Read the model definition and answer for the solid it produces. Units are mm, in the model's axes. A direction names the side the tool comes from. Give positions to 0.01 mm unless a question says otherwise; leave off trailing zeros. Loops run counter-clockwise (first coordinate to the right, second up) from the corner with the lowest first, then second, coordinate; pieces in that order, holes last.
(1) Each of these flat-tipped pins is pushed along its axis until it touches: P1, Ø6.5, axis at y = 0, z = 57, coming from the +X side; P2, Ø1.7, axis at y = 1.5, z = 68.5, coming from the -X side; P3, Ø3, axis at x = 0, z = 4, coming from the +Y side. Where does it stop, or does it pass through?
(2) Determine the mould class of faces 1 (the face through (-2, 2, -77)), 2 (the face through (-3.9, 0, -9)), 3 (the face through (8.201, 4, 1)) for opening direction X: pulls with the +X half, pulls with the -X half, needs draft (parallel to the pull), parting line crosses it, or undercut.
(3) Straight lines are drawn through the part: probe 1 along Y at (x, z) = (0, 72); probe 2 along X at (y, z) = (-3.5, 45); probe 3 along X at (y, z) = (-4.5, 36). For each, find the intervals that lie inside material, in ascending order.
(4) Find section A-A, the plane y = 0. Write down the section's boundary in (x, z), then the cut area to 3 significant figures.
(5) Find section B-B, the plane x = 0. Write down the section's boundary in (y, z).
(6) Which of the six approach directions +Z, -Z, +X, -X, +Y, -Y give full straight-line access (tool end or side, diameter ignored) to faces 4 (the face through (3.9, 0, 67)), 5 (the face through (-3.9, 0, 67)), 6 (the face through (8.201, -4, 1)), 7 (the face through (-10, -7, 1))?
```python
from build123d import *

# Parameters (mm, degrees)
SKETCH1_R               = 2.5
BOSS_EXTRUDE1_DEPTH     = 77
CUT_EXTRUDE1_DEPTH      = 79.880986302
CUT_EXTRUDE1_DEPTH_BACK = 79.880986302
SKETCH2_R               = 2.839339828


with BuildPart() as part:
    # Sketch1 → Boss-Extrude1 (new, symmetric)
    with BuildSketch(Plane.XY):
        Polygon((3.9, -2.839339828), (6.560660172, -5.5), (8.200660172, -5.5), (8.200660172, -3.1), (9.3, -3.1), (10, -3.8), (10, -10), (3.8, -10), (3.1, -9.3), (3.1, -8.200660172), (5.5, -8.200660172), (5.5, -6.560660172), (2.839339828, -3.9), (-2.839339828, -3.9), (-5.5, -6.560660172), (-5.5, -8.200660172), (-3.1, -8.200660172), (-3.1, -9.3), (-3.8, -10), (-10, -10), (-10, -3.8), (-9.3, -3.1), (-8.200660172, -3.1), (-8.200660172, -5.5), (-6.560660172, -5.5), (-3.9, -2.839339828), (-3.9, 2.839339828), (-6.560660172, 5.5), (-8.200660172, 5.5), (-8.200660172, 3.1), (-9.3, 3.1), (-10, 3.8), (-10, 10), (-3.8, 10), (-3.1, 9.3), (-3.1, 8.200660172), (-5.5, 8.200660172), (-5.5, 6.560660172), (-2.839339828, 3.9), (2.839339828, 3.9), (5.5, 6.560660172), (5.5, 8.200660172), (3.1, 8.200660172), (3.1, 9.3), (3.8, 10), (10, 10), (10, 3.8), (9.3, 3.1), (8.200660172, 3.1), (8.200660172, 5.5), (6.560660172, 5.5), (3.9, 2.839339828), align=None)
        Circle(SKETCH1_R, mode=Mode.SUBTRACT)
    extrude(amount=BOSS_EXTRUDE1_DEPTH, both=True)

    # Sketch2 → Cut-Extrude1 (cut, two sides: drawn at the far end of the back side and taken through both)
    with BuildSketch(Plane(origin=(3.9, 0, 0), x_dir=(0, 0, -1), z_dir=(1, 0, 0)).offset(-CUT_EXTRUDE1_DEPTH_BACK)):
        with Locations(Location((-57, 0, 0), (0, 0, 90))):
            Circle(SKETCH2_R)
    extrude(amount=CUT_EXTRUDE1_DEPTH + CUT_EXTRUDE1_DEPTH_BACK, mode=Mode.SUBTRACT)


solid = part.part
```
Entries:
1. P1: stops at x = 9.45
1. P2: stops at x = -3.9
1. P3: stops at y = 3.9
2. face 1: needs draft
2. face 2: pulls with the -X half
2. face 3: undercut
3. probe 1: y = -3.9 to -2.5, 2.5 to 3.9
3. probe 2: x = -9.7 to -8.2, -4.56 to 4.56, 8.2 to 9.7
3. probe 3: x = -10 to -8.2, -5.56 to -3.44, 3.44 to 5.56, 8.2 to 10
4. outline: (-3.9, -77) - (-2.5, -77) - (-2.5, 54.16) - (-3.9, 54.16) - close; (-3.9, 59.84) - (-2.5, 59.84) - (-2.5, 77) - (-3.9, 77) - close; (2.5, -77) - (3.9, -77) - (3.9, 54.16) - (2.5, 54.16) - close; (2.5, 59.84) - (3.9, 59.84) - (3.9, 77) - (2.5, 77) - close
4. area: 415 mm2
5. outline: (-3.9, -77) - (-2.5, -77) - (-2.5, 55.65) arc R2.84 cw to (-2.5, 58.35) - (-2.5, 77) - (-3.9, 77) - close; (2.5, -77) - (3.9, -77) - (3.9, 77) - (2.5, 77) - (2.5, 58.35) arc R2.84 cw to (2.5, 55.65) - close
6. face 4: +Z, -Z, +X
6. face 5: +Z, -Z, -X
6. face 6: +Z, -Z
6. face 7: +Z, -Z, -X, +Y, -Y
